```python
from build123d import *

# Parameters (mm, degrees)
ESQUISSE1_R                  = 20.15
ESQUISSE1_R_2                = 16.15
BOSS_EXTRU_1_DEPTH           = 50
ESQUISSE2_W                  = 10
ESQUISSE2_H                  = 16
BOSS_EXTRU_2_DEPTH           = 20
ENL_V_MAT_EXTRU_1_DEPTH      = 77.302178868
ENL_V_MAT_EXTRU_1_DEPTH_BACK = 77.302178868
ESQUISSE3_R                  = 2.6
CONG_1_R                     = 5
BOSS_EXTRU_3_DEPTH           = 5
BOSS_EXTRU_3_DEPTH_BACK      = 5
ESQUISSE5_W                  = 10
ESQUISSE5_H                  = 6
ESQUISSE4_R                  = 2.25
ENL_V_MAT_EXTRU_2_DEPTH      = 62.684682178
CONG_2_R                     = 3


with BuildPart() as part:
    # Esquisse1 → Boss.-Extru.1 (new body)
    with BuildSketch(Plane.XY):
        Circle(ESQUISSE1_R)
        Circle(ESQUISSE1_R_2, mode=Mode.SUBTRACT)
    extrude(amount=BOSS_EXTRU_1_DEPTH)

    # Esquisse2 → Boss.-Extru.2 (add)
    with BuildSketch(Plane.XY.offset(50)):
        with Locations((-22, 0)):
            Rectangle(ESQUISSE2_W, ESQUISSE2_H)
        with Locations((22, 0)):
            Rectangle(ESQUISSE2_W, ESQUISSE2_H)
    extrude(amount=-BOSS_EXTRU_2_DEPTH)

    # Esquisse3 → Enlèv. mat.-Extru.1 (cut, two sides: drawn at the far end of the back side and taken through both)
    with BuildSketch(Plane.ZY.offset(27).offset(-ENL_V_MAT_EXTRU_1_DEPTH_BACK)):
        with Locations(Location((40, 0, 0), (0, 0, 270))):
            Circle(ESQUISSE3_R)
    extrude(amount=ENL_V_MAT_EXTRU_1_DEPTH + ENL_V_MAT_EXTRU_1_DEPTH_BACK, mode=Mode.SUBTRACT)

    # Congé1
    cong_1_edges = [part.edges().sort_by_distance(p)[0] for p in [
        (22.746925165, 8, 30),
        (22.746925165, -8, 30),
        (22.746925165, 8, 50),
        (22.746925165, -8, 50),
        (-22.746925165, 8, 30),
        (-22.746925165, -8, 30),
        (-22.746925165, 8, 50),
        (-22.746925165, -8, 50),
    ]]
    fillet(cong_1_edges, radius=CONG_1_R)

    # Esquisse5 → Boss.-Extru.3 (add, two sides: drawn at the far end of the back side and taken through both)
    with BuildSketch(Plane(origin=(0, 0, 0), x_dir=(0, 0, -1), z_dir=(1, 0, 0)).offset(-BOSS_EXTRU_3_DEPTH_BACK)):
        with Locations((-8, 21)):
            Rectangle(ESQUISSE5_W, ESQUISSE5_H)
    extrude(amount=BOSS_EXTRU_3_DEPTH + BOSS_EXTRU_3_DEPTH_BACK)

    # Esquisse4 → Enlèv. mat.-Extru.2 (cut, through all)
    with BuildSketch(Plane(origin=(0, 0, 0), x_dir=(1, 0, 0), z_dir=(0, 1, 0))):
        with Locations(Location((0, -8, 0), (0, 0, 90))):
            Circle(ESQUISSE4_R)
    extrude(amount=ENL_V_MAT_EXTRU_2_DEPTH, mode=Mode.SUBTRACT)

    # Congé2
    cong_2_edges = [part.edges().sort_by_distance(p)[0] for p in [
        (5, 21.759898821, 3),
        (5, 21.759898821, 13),
        (-5, 21.759898821, 13),
        (-5, 21.759898821, 3),
    ]]
    fillet(cong_2_edges, radius=CONG_2_R)


solid = part.part
```
Build history of the part. All positions in model axes, mm. A direction names the side the tool comes from. Give positions to 0.01 mm unless a question says otherwise; leave off trailing zeros. Loops run counter-clockwise (first coordinate to the right, second up) from the corner with the lowest first, then second, coordinate; pieces in that order, holes last.
1) Band-saw the part on B-B on z = 40. List the corners of the cut face in (x, y).
Values follow:
outline: (-27, -8) - (-18.49, -8) arc R20.15 ccw to (18.49, -8) - (27, -8) - (27, -2.6) - (15.94, -2.6) arc R16.15 cw to (-15.94, -2.6) - (-27, -2.6) - close; (-27, 2.6) - (-15.94, 2.6) arc R16.15 cw to (15.94, 2.6) - (27, 2.6) - (27, 8) - (18.49, 8) arc R20.15 ccw to (-18.49, 8) - (-27, 8) - close
2) Drop flat-ended pins along their axis: P1, Ø6.5, axis at x = -24, y = 0.5, coming from the -Z side; P2, Ø12, axis at y = 14, z = 18, coming from the -X side; P3, Ø5, axis at x = 18, y = -15.5, coming from the -Z side; P4, Ø9.5, axis at x = 21.5, z = 40, coming from the -Y side. Give the stop position or say it passes through.
Values follow:
P1: stops at z = 30
P2: stops at x = -18.49
P3: passes through
P4: stops at y = -11.2
3) Band-saw the part on D-D on y = 9. List the corners of the cut face in (x, z), then the cut area to 3 significant figures.
Values follow:
outline: (-18.03, 0) - (-13.41, 0) - (-13.41, 50) - (-18.03, 50) - close; (13.41, 0) - (18.03, 0) - (18.03, 50) - (13.41, 50) - close
area: 462 mm2
4) Probe line 1 along X through (y, z) = (22, 8); line 2 along Y through (x, z) = (0, 23.5); line 3 along Y through (x, z) = (21, 40). List the from-to ranges inside material, lowest first.
Values follow:
line 1: x = -5 to -2.25, 2.25 to 5
line 2: y = -20.15 to -16.15, 16.15 to 20.15
line 3: y = -8 to -2.6, 2.6 to 8
5) 3-axis set-ups, long thin cutter, end or side, ignore diameter. For faces 1 (the face through (4.14, 21.79, 3.9)), 2 (the face through (23, -7, 32)), 3 (the face through (-0.099, 19.94, 10.248)), 4 (the face through (-23, 6, 31)): which of +Z, -Z, +X, -X, +Y, -Y reach the whole face in a straight line?
Values follow:
face 1: -Z, +X, +Y
face 2: -Z, +X, -Y
face 3: +Y
face 4: -Z, -X, +Y
6) Band-saw the part on A-A on x = 0. List the corners of the cut face in (y, z).
Values follow:
outline: (-20.15, 0) - (-16.15, 0) - (-16.15, 50) - (-20.15, 50) - close; (16.15, 0) - (20.15, 0) - (20.15, 3) - (24, 3) - (24, 5.75) - (16.15, 5.75) - close; (16.15, 10.25) - (24, 10.25) - (24, 13) - (20.15, 13) - (20.15, 50) - (16.15, 50) - close
7) Two-plate mould, pull along Y, no slides. Class faces 5 (the face through (-21.39, 0.56, 37.46)), 6 (the face through (21.55, 0.56, 37.46)), 7 (the face through (-4.37, -19.67, 24.65)), 8 (the face through (23, 7, 32)): released by +Y, released by -Y, zero draft, split by the parting line, or undercut.
Values follow:
face 5: undercut
face 6: undercut
face 7: split by the parting line
face 8: released by +Y
8) Band-saw the part on C-C on y = 0. List the corners of the cut face in (x, z), then the cut area to 3 significant figures.
Values follow:
outline: (-27, 30) - (-20.15, 30) - (-20.15, 0) - (-16.15, 0) - (-16.15, 37.4) - (-27, 37.4) - close; (-27, 42.6) - (-16.15, 42.6) - (-16.15, 50) - (-27, 50) - close; (16.15, 0) - (20.15, 0) - (20.15, 30) - (27, 30) - (27, 37.4) - (16.15, 37.4) - close; (16.15, 42.6) - (27, 42.6) - (27, 50) - (16.15, 50) - close
area: 561 mm2
